Design review of the part built by this model. Coordinates are the model's own, in mm. Give positions to 0.01 mm unless a question says otherwise; leave off trailing zeros. Order: outer loops, then holes, each group sorted by start corner. A loop starts at its lowest first (then second) coordinate and runs counter-clockwise, first axis right, second up. Notation, with made-up numbers: (-5.5, -9.5) -> (15.5, -9.5) arc R27 cw to (15.5, 25.5) -> close; hole circle Ø9 at (11.25, 83.5). An arc over 180 degrees is marked (long way). Use a Markdown table: item, result. Add a question column.
```python
from build123d import *

# Parameters (mm, degrees)
F0_W     = 190
F0_H     = 20
F1_DEPTH = 1.5
F2_R     = 6
F3_DEPTH = 3.001
F4_R     = 6
F5_DEPTH = 3.001
F6_R     = 9.99999


# Not quite as in the source:
# - a fillet or chamfer is up to 0.001 mm smaller than in the source, because OpenCascade refuses the exact size


with BuildPart() as f1:
    # F0 (on Top) → F1 (new body, symmetric)
    with BuildSketch(Plane.XY):
        Rectangle(F0_W, F0_H)
    extrude(amount=F1_DEPTH, both=True)

    # F2 (on face) → F3 (cut, through all)
    with BuildSketch(Plane.XY.offset(1.5)):
        with Locations((-85, 0)):
            Circle(F2_R)
        with Locations((85, 0)):
            Circle(F2_R)
    extrude(amount=-F3_DEPTH, mode=Mode.SUBTRACT)

    # F4 (on face) → F5 (cut, through all)
    with BuildSketch(Plane.XY.offset(1.5)):
        Circle(F4_R)
    extrude(amount=-F5_DEPTH, mode=Mode.SUBTRACT)

    # F6 (radius 10 in the source; OpenCascade refuses exactly that, so slightly less here)
    f6_edges = [f1.edges().sort_by_distance(p)[0] for p in [
        (-95, -10, 0),
        (-95, 10, 0),
        (95, -10, 0),
        (95, 10, 0),
    ]]
    fillet(f6_edges, radius=F6_R)


solid = f1.part
```
1) Add section C-C (y = -3.75). Give the boundary of the cut face in (x, z).
2) Add section B-B (z = -0.55). Give the number of separate pieces and of enclosed holes in the cut face, then the cut area to 3 significant figures.
3) Add section A-A (x = 0). Give the boundary of the cut face in (y, z), then the cut area to 3 significant figures.
4) The part is to be moulded in two halves that separate along Y. For faces 1 (the cylindrical face through (91.99, 7.15, -0.02)), 2 (the flat face through (-1, 7, 1.5)), 3 (the cylindrical face through (79, 0, 0)), say which applies: +Y half, -Y half, draft (parallel to the pull), parting line (faces both ways), or undercut.
5) Insertion check: pin 1 (9.5 mm diameter, centred on x = 0, y = 0, fed in from +Z). The pin has a flat end and moves straight along its axis. Give the tip position at first contact, or say it passes through.
6) For L1, parallel to X at y = -4.5, z = -0.8; L2, parallel to Y at x = -85, z = -0.65; L3, parallel to X at y = -5.5, z = -0.85, list the stretches that pass through material, from the lowest coordinate up. Write a range as [from, to].
Worked answers:
| question | item | result |
|---|---|---|
| 1 | outline | (-94.27, -1.5) -> (-89.68, -1.5) -> (-89.68, 1.5) -> (-94.27, 1.5) -> close; (-80.32, -1.5) -> (-4.68, -1.5) -> (-4.68, 1.5) -> (-80.32, 1.5) -> close; (4.68, -1.5) -> (80.32, -1.5) -> (80.32, 1.5) -> (4.68, 1.5) -> close; (89.68, -1.5) -> (94.27, -1.5) -> (94.27, 1.5) -> (89.68, 1.5) -> close |
| 2 | separate pieces | 1 |
| 2 | enclosed holes | 3 |
| 2 | area | 3,370 mm^2 |
| 3 | outline | (-10, -1.5) -> (-6, -1.5) -> (-6, 1.5) -> (-10, 1.5) -> close; (6, -1.5) -> (10, -1.5) -> (10, 1.5) -> (6, 1.5) -> close |
| 3 | area | 24.0 mm^2 |
| 4 | face 1 | +Y half |
| 4 | face 2 | draft |
| 4 | face 3 | undercut |
| 5 | pin 1 | through |
| 6 | L1 | [-93.93, -88.97], [-81.03, -3.97], [3.97, 81.03], [88.97, 93.93] |
| 6 | L2 | [-10, -6], [6, 10] |
| 6 | L3 | [-93.35, -87.4], [-82.6, -2.4], [2.4, 82.6], [87.4, 93.35] |
